Geometry check sheet. Reference: the model listing, model coordinates, mm. Face numbers are marked on the shaded views. Round coordinates to 2 decimals unless told otherwise and drop trailing zeros. Loops run counter-clockwise (first coordinate to the right, second up) from the corner with the lowest first, then second, coordinate; pieces in that order, holes last. Notation, with made-up numbers: (-19, 14.25) - (-8, 14.25) arc R12 cw to (-8, 27.25) - close; hole circle Ø9 at (13.25, -4). An arc over 180 degrees is marked (long way). Write item = value, one per line.
```python
from build123d import *

# Parameters (mm, degrees)
PANEL_DEPTH        = 3
INSERT_DEPTH       = 3
SKETCH3_W          = 15
SKETCH3_H          = 7
CUT_EXTRUDE1_DEPTH = 256.411638929


with BuildPart() as part:
    # Sketch1 → panel (new body)
    with BuildSketch(Plane.XY):
        Polygon((-232.020441826, 85.609661267), (-232.020441826, 101.609661267), (-227.020441826, 106.609661267), (-179.020441826, 106.609661267), (-174.020441826, 101.609661267), (-174.020441826, 85.609661267), (-179.020441826, 80.609661267), (-227.020441826, 80.609661267), align=None)
    extrude(amount=PANEL_DEPTH)

    # Sketch2 → insert (add)
    with BuildSketch(Plane(origin=(0, 0, 3), x_dir=(-1, 0, 0), z_dir=(0, 0, -1))):
        Polygon((176.120441826, 86.479509748), (176.120441826, 100.739812786), (179.890290307, 104.509661267), (226.150593345, 104.509661267), (229.920441826, 100.739812786), (229.920441826, 86.479509748), (226.150593345, 82.709661267), (179.890290307, 82.709661267), align=None)
    extrude(amount=-INSERT_DEPTH)

    # Sketch3 → Cut-Extrude1 (cut, through all)
    with BuildSketch(Plane.XY):
        with Locations((-203.020441826, 84.109661267)):
            Rectangle(SKETCH3_W, SKETCH3_H)
    extrude(amount=CUT_EXTRUDE1_DEPTH, mode=Mode.SUBTRACT)


solid = part.part
```
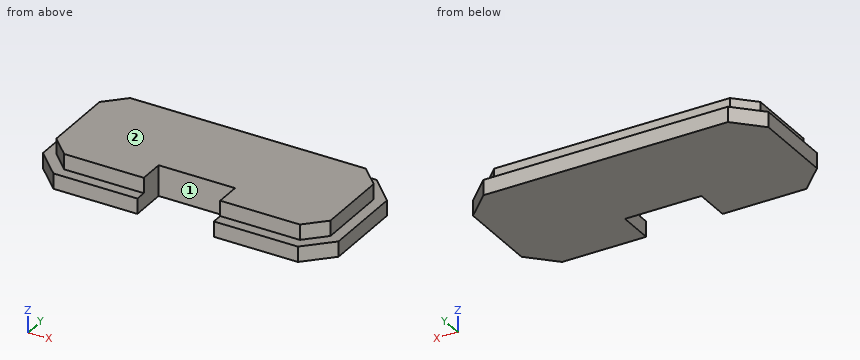
(1) Gauge pin test, flat ends, axial feed: pin 1 (1.5 mm diameter, centred on y = 97, z = 4, fed in from -X); pin 2 (0.9 mm diameter, centred on x = -202.5, z = 4.5, fed in from +Y); pin 3 (3 mm diameter, centred on y = 82.5, z = 3.5, fed in from +X). Record the tip position at first contact, or that the pin passes through.
Answers follow:
pin_1 = -229.92
pin_2 = 104.51
pin_3 = -175.72
(2) Section check C-C (x = -186). Enter the section's corners in (y, z), then the cut area to 3 significant figures.
Answers follow:
outline = (80.61, 0) - (106.61, 0) - (106.61, 3) - (104.51, 3) - (104.51, 6) - (82.71, 6) - (82.71, 3) - (80.61, 3) - close
area = 143 mm²
(3) Section check D-D (z = 0.75). Enter the section's corners in (x, y).
Answers follow:
outline = (-232.02, 85.61) - (-227.02, 80.61) - (-210.52, 80.61) - (-210.52, 87.61) - (-195.52, 87.61) - (-195.52, 80.61) - (-179.02, 80.61) - (-174.02, 85.61) - (-174.02, 101.61) - (-179.02, 106.61) - (-227.02, 106.61) - (-232.02, 101.61) - close
(4) Section check B-B (z = 4). Enter the section's corners in (x, y).
Answers follow:
outline = (-229.92, 86.48) - (-226.15, 82.71) - (-210.52, 82.71) - (-210.52, 87.61) - (-195.52, 87.61) - (-195.52, 82.71) - (-179.89, 82.71) - (-176.12, 86.48) - (-176.12, 100.74) - (-179.89, 104.51) - (-226.15, 104.51) - (-229.92, 100.74) - close
(5) Mould release check, pull along X, two halves, no side actions. Record for the marked faces 1 and 2: pulls with the +X half, pulls with the -X half, needs draft (parallel to the pull), parting line crosses it, or undercut.
Answers follow:
face_1 = undercut
face_2 = needs draft
(6) Section check A-A (y = 95). Enter the section's corners in (x, z), then the cut area to 3 significant figures.
Answers follow:
outline = (-232.02, 0) - (-174.02, 0) - (-174.02, 3) - (-176.12, 3) - (-176.12, 6) - (-229.92, 6) - (-229.92, 3) - (-232.02, 3) - close
area = 335 mm²
(7) Scan lines: L1, parallel to X at y = 87.5, z = 4.1; L2, parallel to Y at x = -225.5, z = 5.05; L3, parallel to Z at x = -187, y = 104.75. Record each from-to range of solid material in increasing order. Write a range as [from, to].
Answers follow:
L1 = [-229.92, -210.52], [-195.52, -176.12]
L2 = [82.71, 104.51]
L3 = [0, 3]
